For this review, take the finished solid that the model builds, in its own axes (mm). A direction names the side the tool comes from. Coordinates: 2 decimals unless noted, no trailing zeros. Order: outer loops, then holes, each group sorted by start corner. A loop starts at its lowest first (then second) coordinate and runs counter-clockwise, first axis right, second up.
from build123d import *

# Parameters (mm, degrees)
SKETCH1_R           = 2
SKETCH1_R_2         = 1.25
SKETCH1_W           = 23.5
SKETCH1_H           = 13
BOSS_EXTRUDE1_DEPTH = 4
SKETCH3_R           = 10
BOSS_EXTRUDE2_DEPTH = 7
SKETCH4_R           = 8.5
CUT_EXTRUDE1_DEPTH  = 3


with BuildPart() as part:
    # Sketch1 → Boss-Extrude1 (new body)
    with BuildSketch(Plane.XY):
        with BuildLine():
            Line((-9, 12.5), (-2.401010284, 19.772380391))
            ThreePointArc((-2.401010284, 19.772380391), (0, 20.766911414), (2.401010284, 19.772380391))
            Line((2.401010284, 19.772380391), (9, 12.5))
            Line((9, 12.5), (17.5, 12.5))
            ThreePointArc((17.5, 12.5), (30, 0), (17.5, -12.5))
            Line((17.5, -12.5), (9, -12.5))
            Line((9, -12.5), (2.401010284, -19.772380391))
            ThreePointArc((2.401010284, -19.772380391), (0, -20.766911414), (-2.401010284, -19.772380391))
            Line((-2.401010284, -19.772380391), (-9, -12.5))
            Line((-9, -12.5), (-17.5, -12.5))
            ThreePointArc((-17.5, -12.5), (-30, 0), (-17.5, 12.5))
            Line((-17.5, 12.5), (-9, 12.5))
        make_face()
        with Locations((0, 16.5)):
            Circle(SKETCH1_R, mode=Mode.SUBTRACT)
        with Locations(Location((0, -16.5, 0), (0, 0, 180))):
            Circle(SKETCH1_R, mode=Mode.SUBTRACT)
        with Locations((-3, 0)):
            Circle(SKETCH1_R_2, mode=Mode.SUBTRACT)
        with Locations((24.5, 0)):
            Circle(SKETCH1_R_2, mode=Mode.SUBTRACT)
        with Locations((10.75, 0)):
            Rectangle(SKETCH1_W, SKETCH1_H, mode=Mode.SUBTRACT)
    extrude(amount=BOSS_EXTRUDE1_DEPTH)

    # Sketch3 → Boss-Extrude2 (add)
    with BuildSketch(Plane.XY.offset(4)):
        with Locations((-15.3, 0)):
            Circle(SKETCH3_R)
    extrude(amount=BOSS_EXTRUDE2_DEPTH)

    # Sketch4 → Cut-Extrude1 (cut)
    with BuildSketch(Plane.XY.offset(11)):
        with Locations((-15.35, 0)):
            Circle(SKETCH4_R)
    extrude(amount=-CUT_EXTRUDE1_DEPTH, mode=Mode.SUBTRACT)


solid = part.part
1. To check wall thickness, follow L1, parallel to Y at x = -15.35, z = 9.95; L2, parallel to Y at x = 0, z = 1.4; L3, parallel to Y at x = -1.5, z = 3.75. State the ranges of each line that lie inside material, in increasing order.
Answer below:
L1: y = -10 to -8.5, 8.5 to 10
L2: y = -20.77 to -18.5, -14.5 to -6.5, 6.5 to 14.5, 18.5 to 20.77
L3: y = -20.42 to -17.82, -15.18 to 15.18, 17.82 to 20.42
2. Clearance check with flat-ended pins moving along their axes: pin 1 Ø4.5 at (x, z) = (-12.5, 1) entering from -Y; pin 2 Ø12 at (x, y) = (13, 2.5) entering from +Z; pin 3 Ø2 at (x, y) = (24.5, 0) entering from +Z; pin 4 Ø1.2 at (y, z) = (-3, 2) entering from +X. State where each tip first meets the part, or that it passes through.
Answer below:
pin 1: stops at y = -12.5
pin 2: stops at z = 4
pin 3: passes through
pin 4: stops at x = 29.77
3. Take a section at C-C, the plane y = 16.5. Give the boundary of the cut face in (x, z), plus the area to 3 significant figures.
Answer below:
outline: (-5.37, 0) - (-2, 0) - (-2, 4) - (-5.37, 4) - close; (2, 0) - (5.37, 0) - (5.37, 4) - (2, 4) - close
area: 27.0 mm2
4. Take a section at B-B, the plane z = 3. Give the boundary of the cut face in (x, y), plus the area to 3 significant figures.
Answer below:
outline: (-17.5, -12.5) - (-9, -12.5) - (-2.4, -19.77) arc R3.4 ccw to (2.4, -19.77) - (9, -12.5) - (17.5, -12.5) arc R12.5 ccw to (17.5, 12.5) - (9, 12.5) - (2.4, 19.77) arc R3.4 ccw to (-2.4, 19.77) - (-9, 12.5) - (-17.5, 12.5) arc R12.5 ccw to start; hole circle Ø2.5 at (-3, 0); hole circle Ø4 at (0, -16.5); hole circle Ø4 at (0, 16.5); hole (-1, -6.5) - (22.5, -6.5) - (22.5, 6.5) - (-1, 6.5) - close; hole circle Ø2.5 at (24.5, 0)
area: 1,200 mm2
5. Take a section at D-D, the plane x = 24.5. Give the boundary of the cut face in (y, z).
Answer below:
outline: (-10.36, 0) - (-1.25, 0) - (-1.25, 4) - (-10.36, 4) - close; (1.25, 0) - (10.36, 0) - (10.36, 4) - (1.25, 4) - close
6. Take a section at A-A, the plane y = 0. Give the boundary of the cut face in (x, z).
Answer below:
outline: (-30, 0) - (-4.25, 0) - (-4.25, 4) - (-5.3, 4) - (-5.3, 11) - (-6.85, 11) - (-6.85, 8) - (-23.85, 8) - (-23.85, 11) - (-25.3, 11) - (-25.3, 4) - (-30, 4) - close; (-1.75, 0) - (-1, 0) - (-1, 4) - (-1.75, 4) - close; (22.5, 0) - (23.25, 0) - (23.25, 4) - (22.5, 4) - close; (25.75, 0) - (30, 0) - (30, 4) - (25.75, 4) - close
7. Machinability: for faces 1 (the face through (-6, 0, 0)), 2 (the face through (11, 6.5, 2)), 3 (the face through (-5.65, -16.19, 1.97)), 4 (the face through (13, -12.5, 2)), 5 (the face through (13, 12.5, 2)), which of the approach directions +Z, -Z, +X, -X, +Y, -Y give a long, thin tool a straight path to every point of the face, cutting with its end or side? Answer none if there is none.
Answer below:
face 1: -Z, +X, -X, +Y, -Y
face 2: +Z, -Z
face 3: +Z, -Z, -X, -Y
face 4: +Z, -Z, +X, -Y
face 5: +Z, -Z, +X, +Y
8. The part is to be moulded in two halves that separate along Y. For faces 6 (the face through (-13, 12.5, 2)), 7 (the face through (-13, -12.5, 2)), 8 (the face through (22.5, 0, 2)), say which applies: +Y half, -Y half, draft (parallel to the pull), parting line (faces both ways), or undercut.
Answer below:
face 6: +Y half
face 7: -Y half
face 8: undercut
